```python
from build123d import *

# Parameters (mm, degrees)
EXTRUDE_1_DEPTH      = 300
FILLET_1_R           = 10
SHELL_START          = -298
SHELL_1_DEPTH        = 296
SKETCH_2_R           = 4
CUT_EXTRUDE_1_DEPTH  = 649.459713475
EXTRUDE_2_DEPTH      = 300
CUT_EXTRUDE_12_DEPTH = 10


# Read off the part's stored shape, not the designer's step: 抽壳1
with BuildPart() as part:
    # 草图1 → 凸台-拉伸1 (new body)
    with BuildSketch(Plane.XY):
        with BuildLine():
            Line((440, -20), (440, 0))
            Line((440, 0), (90, 0))
            Line((90, 0), (90, 300))
            ThreePointArc((90, 300), (22.32945557, 369.961229526), (-49.84496105, 304.656330737))
            Line((-49.84496105, 304.656330737), (-89.800664207, 5.986710947))
            ThreePointArc((-89.800664207, 5.986710947), (-89.720985624, -7.081294982), (-87.749643874, -20))
            Line((-87.749643874, -20), (0, -20))
            Line((0, -20), (400, -20))
            Line((400, -20), (440, -20))
        make_face()
    extrude(amount=-EXTRUDE_1_DEPTH)

    # 圆角1
    fillet_1_edges = [part.edges().sort_by_distance(p)[0] for p in [
        (440, 0, -150),
    ]]
    fillet(fillet_1_edges, radius=FILLET_1_R)

    # 抽壳1 outline → 抽壳1 (cut)
    with BuildSketch(Plane.XY.offset(SHELL_START)):
        with BuildLine():
            Line((88, -2), (88, 300))
            ThreePointArc((88, 300), (22.229935395, 367.963426842), (-47.85374671, 304.45747209))
            Line((-47.85374671, 304.45747209), (-87.809464232, 5.787744921))
            ThreePointArc((-87.809464232, 5.787744921), (-87.706256756, -7.184185814), (-85.697141143, -20))
            Line((-85.697141143, -20), (438, -20))
            Line((438, -20), (438, -10))
            ThreePointArc((438, -10), (435.656854249, -4.343145751), (430, -2))
            Line((430, -2), (88, -2))
        make_face()
    extrude(amount=SHELL_1_DEPTH, mode=Mode.SUBTRACT)

    # 草图2 → 切除-拉伸1 (cut, through all)
    with BuildSketch(Plane.XY):
        Circle(SKETCH_2_R)
        with Locations((20, 300)):
            Circle(SKETCH_2_R)
    extrude(amount=-CUT_EXTRUDE_1_DEPTH, mode=Mode.SUBTRACT)

    # 草图3 → 凸台-拉伸2 (add)
    with BuildSketch(Plane.XY):
        with BuildLine():
            Line((88.022724339, 0), (90, 0))
            ThreePointArc((90, 0), (89.435641521, -10.063102189), (87.749643874, -20))
            Line((87.749643874, -20), (85.720475967, -20))
            ThreePointArc((85.720475967, -20), (87.4452681, -10.066036305), (88.022724339, 0))
        make_face()
    extrude(amount=-EXTRUDE_2_DEPTH)

    # 草图4 → 切除-拉伸12 (cut)
    with BuildSketch(Plane.ZY.offset(-88)):
        Polygon((-7, 231), (-3, 231), (-3, 299), (-7, 299), (-293, 299), (-297, 299), (-297, 231), align=None)
    extrude(amount=-CUT_EXTRUDE_12_DEPTH, mode=Mode.SUBTRACT)


solid = part.part
```
Model file for the job. Use its own axes, mm. A direction names the side the tool comes from. Give positions to 0.01 mm unless a question says otherwise; leave off trailing zeros. Write each loop counter-clockwise with the first axis right and the second up, starting at its lowest first coordinate (ties: lowest second). Pieces come first, ordered by that corner, then holes. Notation, with made-up numbers: (-14, -34.5) -> (28, -34.5) arc R21 cw to (28, -10.5) -> close; hole circle Ø2 at (-6, -39). An arc over 180 degrees is marked (long way). Use CSV: the item, a comma, the result in double quotes. Start each with the question number.
1) Cut at D-D on x = 10. List the corners of the cut face in (y, z).
2) Pin check, flat tips, straight feed: P1, Ø4, axis at x = 182, z = -54, coming from the +Y side; P2, Ø5, axis at y = -14.5, z = -166, coming from the -X side; P3, Ø10, axis at y = 253.5, z = -266, coming from the -X side. Stop position of each tip, or through.
3) Cut at A-A on z = -139. List the corners of the cut face in (x, y).
4) Cut at C-C on y = 244.5. List the corners of the cut face in (x, z).
5) Two-plate mould, pull along X, no slides. Class faces 5 (the cylindrical face through (23.835, 369.895, -147.9)), 6 (the cylindrical face through (-87.72, -7, -152.07)), 7 (the flat face through (36, 133, 0)): released by +X, released by -X, zero draft, split by the parting line, or undercut.
6) Drill centre lines: L1, parallel to Z at x = 16.5, y = 76.5; L2, parallel to X at y = 6.5, z = -83; L3, parallel to Y at x = 20, z = -0.45. Where is each one in solid material? Low to high.
7) Tool access for faces 1 (the cylindrical face through (87.31, -11.19, -147.93)), 2 (the flat face through (90, 115, -148)), 3 (the flat face through (260, -11, -298)), 4 (the flat face through (36, 133, -300)): list every direction of +Z, -Z, +X, -X, +Y, -Y with a clear straight run to the whole face (end or side of a thin tool).
8) Cut at B-B on x = 177. List the corners of the cut face in (y, z), plus the area to 3 significant figures.
Final values:
1,outline,"(-20, -300) -> (369.28, -300) -> (369.28, 0) -> (-20, 0) -> (-20, -2) -> (367.26, -2) -> (367.26, -298) -> (-20, -298) -> close"
2,P1,"stops at y = 0"
2,P2,"stops at x = -89.2"
2,P3,"stops at x = -57.36"
3,outline,"(-89.8, 5.99) arc R90 ccw to (-87.75, -20) -> (-85.7, -20) arc R88 cw to (-87.81, 5.79) -> (-47.85, 304.46) arc R68 cw to (88, 300) -> (88, 299) -> (90, 299) -> (90, 300) arc R70 ccw to (-49.84, 304.66) -> close; (85.72, -20) -> (87.75, -20) arc R90 ccw to (89.98, -2) -> (430, -2) arc R8 cw to (438, -10) -> (438, -20) -> (440, -20) -> (440, -10) arc R10 ccw to (430, 0) -> (90, 0) -> (90, 231) -> (88, 231) -> (88, -2) arc R88.02 cw to start"
4,outline,"(-57.89, -300) -> (90, -300) -> (90, -297) -> (88, -297) -> (88, -298) -> (-55.87, -298) -> (-55.87, -2) -> (88, -2) -> (88, -3) -> (90, -3) -> (90, 0) -> (-57.89, 0) -> close"
5,face 5,"split by the parting line"
5,face 6,"undercut"
5,face 7,"zero draft"
6,L1,"z = -300 to -298, -2 to 0"
6,L2,"x = -89.73 to -87.71, 88 to 90"
6,L3,"y = -20 to 296, 304 to 370"
7,face 1,"none"
7,face 2,"+Z, -Z, +X, +Y"
7,face 3,"-Y"
7,face 4,"-Z, +X, -X, +Y, -Y"
8,outline,"(-20, -300) -> (0, -300) -> (0, 0) -> (-20, 0) -> (-20, -2) -> (-2, -2) -> (-2, -298) -> (-20, -298) -> close"
8,area,"672 mm2"
